Source: CAD feature listing. Evaluate the final solid. Frame: model axes, mm. A direction names the side the tool comes from. Coordinates: 2 decimals unless noted, no trailing zeros. Order: outer loops, then holes, each group sorted by start corner. A loop starts at its lowest first (then second) coordinate and runs counter-clockwise, first axis right, second up. Notation, with made-up numbers: (47, 58) -> (79, 58) arc R19 ccw to (79, 73) -> close; hole circle Ø4 at (46.5, 0). An arc over 180 degrees is marked (long way). Write item = value, one per line. Start each with the question number.
Item 1: Section query C-C (z = -29). Output: boundary loops of the cut face in (x, y).
Item 2: Mould query, pull axis X, two halves, no side actions, for faces 1 (the cylindrical face through (-45.34, 4.93, 62.85)), 2 (the cylindrical face through (73.625, 4.93, -24.194)), 3 (the flat face through (-16, 10, 9)), 4 (the cylindrical face through (-73.785, 4.93, -23.703)). Classes: released by +X, released by -X, zero draft, split by the parting line, or undercut.
Item 3: Section query A-A (y = 1.75). Output: boundary loops of the cut face in (x, z), then the cut area to 3 significant figures.
Item 4: Ray query, line 1 along Z through (x, y) = (0, 7); line 2 along X through (y, z) = (8.5, 52.5); line 3 along Z through (x, y) = (0.5, 2). Return the intervals inside material, ascending. Write a range as [from, to].
Item 5: Set-up query: faces 5 (the cylindrical face through (51.666, 4.93, 16.345)), 6 (the flat face through (0, 5, 17.5)). Return all of +Z, -Z, +X, -X, +Y, -Y with unobstructed straight access to the full face (end or side cutting, diameter ignored); none if empty.
Item 6: Section query B-B (z = -62.5). Output: boundary loops of the cut face in (x, y).
Item 7: Contact query for flat-ended pins moving along their axis: pin 1 (2 mm diameter, centred on y = 2.5, z = 33.5, fed in from +X); pin 2 (2 mm diameter, centred on y = 6, z = 46.5, fed in from +X); pin 3 (1 mm diameter, centred on x = -44, y = 5, fed in from -Z). Output: stop coordinate, or through.
```python
from build123d import *

# Parameters (mm, degrees)
SKETCH1_R           = 8
BOSS_EXTRUDE3_DEPTH = 10


with BuildPart() as part:
    # Sketch1 → Boss-Extrude3 (new body)
    with BuildSketch(Plane(origin=(0, 0, 0), x_dir=(1, 0, 0), z_dir=(0, 1, 0))):
        with BuildLine():
            ThreePointArc((14.132148934, 67.528157367), (31.850049433, 43.837832205), (59.85601991, 34.307820558))
            ThreePointArc((59.85601991, 34.307820558), (73.706880013, 23.948817064), (68.590168285, 7.426875892))
            ThreePointArc((68.590168285, 7.426875892), (51.534462525, -16.744561909), (51.125203669, -46.324758182))
            ThreePointArc((51.125203669, -46.324758182), (45.553357053, -62.698817064), (28.25890636, -62.938095635))
            ThreePointArc((28.25890636, -62.938095635), (0, -54.186540592), (-28.25890636, -62.938095635))
            ThreePointArc((-28.25890636, -62.938095635), (-45.553357053, -62.698817064), (-51.125203669, -46.324758182))
            ThreePointArc((-51.125203669, -46.324758182), (-51.534462525, -16.744561909), (-68.590168285, 7.426875892))
            ThreePointArc((-68.590168285, 7.426875892), (-73.706880013, 23.948817064), (-59.85601991, 34.307820558))
            ThreePointArc((-59.85601991, 34.307820558), (-31.850049433, 43.837832205), (-14.132148934, 67.528157367))
            ThreePointArc((-14.132148934, 67.528157367), (0, 77.5), (14.132148934, 67.528157367))
        make_face()
        with Locations((36.736578268, -50.563562148)):
            Circle(SKETCH1_R, mode=Mode.SUBTRACT)
        with Locations((-36.736578268, -50.563562148)):
            Circle(SKETCH1_R, mode=Mode.SUBTRACT)
        with Locations((59.441032268, 19.313562148)):
            Circle(SKETCH1_R, mode=Mode.SUBTRACT)
        with Locations((-59.441032268, 19.313562148)):
            Circle(SKETCH1_R, mode=Mode.SUBTRACT)
        with Locations((0, 62.5)):
            Circle(SKETCH1_R, mode=Mode.SUBTRACT)
        Polygon((20.57248383, 6.684405197), (0, 21.631189606), (-20.57248383, 6.684405197), (-12.71449424, -17.5), (12.71449424, -17.5), align=None, mode=Mode.SUBTRACT)
    extrude(amount=BOSS_EXTRUDE3_DEPTH)


solid = part.part
```
Computed:
q1.outline = (-70.89, 0) -> (70.89, 0) -> (70.89, 10) -> (-70.89, 10) -> close
q2.face_1 = undercut
q2.face_2 = released by +X
q2.face_3 = zero draft
q2.face_4 = released by -X
q3.outline = (-68.59, -7.43) arc R15 ccw to (-59.86, -34.31) arc R50 cw to (-14.13, -67.53) arc R15 ccw to (14.13, -67.53) arc R50 cw to (59.86, -34.31) arc R15 ccw to (68.59, -7.43) arc R50 cw to (51.13, 46.32) arc R15 ccw to (28.26, 62.94) arc R50 cw to (-28.26, 62.94) arc R15 ccw to (-51.13, 46.32) arc R50 cw to start; hole circle Ø16 at (-59.44, -19.31); hole circle Ø16 at (-36.74, 50.56); hole (-20.57, -6.68) -> (0, -21.63) -> (20.57, -6.68) -> (12.71, 17.5) -> (-12.71, 17.5) -> close; hole circle Ø16 at (0, -62.5); hole circle Ø16 at (36.74, 50.56); hole circle Ø16 at (59.44, -19.31)
q3.area = 10,900 mm^2
q4.line_1 = [-77.5, -70.5], [-54.5, -21.63], [17.5, 54.19]
q4.line_2 = [-51.61, -44.5], [-28.97, 28.97], [44.5, 51.61]
q4.line_3 = [-77.49, -70.48], [-54.52, -21.27], [17.5, 54.19]
q5.face_5 = +X, +Y, -Y
q5.face_6 = +Y, -Y
q6.outline = (-16.24, 0) -> (-8, 0) -> (-8, 10) -> (-16.24, 10) -> close; (8, 0) -> (16.24, 0) -> (16.24, 10) -> (8, 10) -> close
q7.pin_1 = 49.14
q7.pin_2 = 51.42
q7.pin_3 = -37.54
